```python
from build123d import *

# Parameters (mm, degrees)
BOX_W               = 14
BOX_H               = 10
BOX_DEPTH           = 20
BOX_PLACEMENT_ANGLE = 157
SKETCH_W            = 40
SKETCH_H            = 40
SKETCH_R            = 1.8
SKETCH_R_2          = 10
PAD_DEPTH           = 10
SKETCH001_R         = 11.05
POCKET_DEPTH        = 7


with BuildPart() as cube:
    # Box → Box (new body)
    with BuildSketch(Plane.XY):
        with Locations((7, 5)):
            Rectangle(BOX_W, BOX_H)
    extrude(amount=BOX_DEPTH)


with BuildPart() as cube_1:
    # Box placement: moved
    add(cube.part.moved(Location((-7, -11, 11))).rotate(Axis((-7, -11, 11), (1, 0, 0)), BOX_PLACEMENT_ANGLE))


with BuildPart() as cut:
    # Sketch → Pad (new body)
    with BuildSketch(Plane.XY):
        Rectangle(SKETCH_W, SKETCH_H)
        with Locations((-15.5, 15.5)):
            Circle(SKETCH_R, mode=Mode.SUBTRACT)
        with Locations((15.5, 15.5)):
            Circle(SKETCH_R, mode=Mode.SUBTRACT)
        with Locations((-15.5, -15.5)):
            Circle(SKETCH_R, mode=Mode.SUBTRACT)
        with Locations((15.5, -15.5)):
            Circle(SKETCH_R, mode=Mode.SUBTRACT)
        Circle(SKETCH_R_2, mode=Mode.SUBTRACT)
    extrude(amount=PAD_DEPTH)

    # Sketch001 → Pocket (cut)
    with BuildSketch(Plane.XY.offset(10)):
        Circle(SKETCH001_R)
    extrude(amount=-POCKET_DEPTH, mode=Mode.SUBTRACT)

    # Cut: cut Cube
    add(cube_1.part, mode=Mode.SUBTRACT)


solid = cut.part
```
Input: part model. Units: mm. Frame: model coordinates. A direction names the side the tool comes from. Give positions to 0.01 mm unless a question says otherwise; leave off trailing zeros. Loops run counter-clockwise (first coordinate to the right, second up) from the corner with the lowest first, then second, coordinate; pieces in that order, holes last.
1) Line query: L1, parallel to Y at x = -15.5, z = 2; L2, parallel to X at y = 0, z = 1.15; L3, parallel to X at y = 15, z = 7.25. Output: solid intervals per line, ascending.
A:
L1: y = -20 to -17.3, -13.7 to 13.7, 17.3 to 20
L2: x = -20 to -10, 10 to 20
L3: x = -20 to -17.23, -13.77 to 13.77, 17.23 to 20
2) Contact query for flat-ended pins moving along their axis: pin 1 (11 mm diameter, centred on x = 4.5, y = -2.5, fed in from +Z); pin 2 (1.5 mm diameter, centred on x = 4, z = 4.5, fed in from -Y). Output: stop coordinate, or through.
A:
pin 1: stops at z = 3
pin 2: stops at y = -14.08
3) Reachability of faces 1 (the cylindrical face through (-2.395, -10.787, 6.549)), 2 (the flat face through (-7, -17, 5)), 3 (the flat face through (9, 9, 10)) from +Z, -Z, +X, -X, +Y, -Y: full face, straight path, thin tool, end or side. Return the list, or none.
A:
face 1: +Z
face 2: +Z, -Y
face 3: +Z, +X, -X, +Y, -Y
4) Section query A-A on y = 15.5. Return the cut outline in (x, z).
A:
outline: (-20, 0) - (-17.3, 0) - (-17.3, 10) - (-20, 10) - close; (-13.7, 0) - (13.7, 0) - (13.7, 10) - (-13.7, 10) - close; (17.3, 0) - (20, 0) - (20, 10) - (17.3, 10) - close
5) Section query C-C on y = 0. Return the cut outline in (x, z).
A:
outline: (-20, 0) - (-10, 0) - (-10, 3) - (-11.05, 3) - (-11.05, 10) - (-20, 10) - close; (10, 0) - (20, 0) - (20, 10) - (11.05, 10) - (11.05, 3) - (10, 3) - close
6) Section query D-D on z = 1. Return the cut outline in (x, y), and give its area (3 significant figures).
A:
outline: (-20, -20) - (-7, -20) - (-7, -15.24) - (7, -15.24) - (7, -20) - (20, -20) - (20, 20) - (-20, 20) - close; hole circle Ø3.6 at (-15.5, -15.5); hole circle Ø3.6 at (-15.5, 15.5); hole circle Ø20 at (0, 0); hole circle Ø3.6 at (15.5, -15.5); hole circle Ø3.6 at (15.5, 15.5)
area: 1,180 mm2
